For this review, take the finished solid that the model builds, in its own axes (mm). A direction names the side the tool comes from. Round coordinates to 2 decimals unless told otherwise and drop trailing zeros. Write each loop counter-clockwise with the first axis right and the second up, starting at its lowest first coordinate (ties: lowest second). Pieces come first, ordered by that corner, then holes. Notation, with made-up numbers: (63, 1.5) -> (94, 1.5) arc R23 cw to (94, 24.5) -> close; hole circle Ø5 at (66, 72). An arc over 180 degrees is marked (long way). Answer in a Markdown table with one row per item. Add a question column.
```python
from build123d import *

# Parameters (mm, degrees)
F0_R     = 4.25
F0_R_2   = 2.6
F1_DEPTH = 8
F0_R_3   = 10.25
F0_R_4   = 1.6
F2_DEPTH = 8
F3_DEPTH = 8
F4_DEPTH = 8
F5_R     = 1.9
F6_DEPTH = 27


with BuildPart() as f1:
    # F0 (on Top) → F1 (new body)
    with BuildSketch(Plane.XY):
        Circle(F0_R)
        Circle(F0_R_2, mode=Mode.SUBTRACT)
    extrude(amount=F1_DEPTH)

    # F0 (on Top) → F2 (join)
    with BuildSketch(Plane.XY):
        Circle(F0_R_3)
        with Locations((0, -7)):
            Circle(F0_R_2, mode=Mode.SUBTRACT)
        with Locations((-7, 0)):
            Circle(F0_R_4, mode=Mode.SUBTRACT)
        with Locations((-4.95, 4.9494949237)):
            Circle(F0_R_4, mode=Mode.SUBTRACT)
        Circle(F0_R, mode=Mode.SUBTRACT)
        with Locations((7, 0)):
            Circle(F0_R_4, mode=Mode.SUBTRACT)
        with Locations((4.95, 4.9494949237)):
            Circle(F0_R_4, mode=Mode.SUBTRACT)
        with Locations((0, 7)):
            Circle(F0_R_4, mode=Mode.SUBTRACT)
    extrude(amount=F2_DEPTH)

    # F0 (on Top) → F3 (join)
    with BuildSketch(Plane.XY):
        with BuildLine():
            ThreePointArc((11.5318049333, -3.3192581973), (11.8823747458, -1.6760579943), (12, 0))
            ThreePointArc((12, 0), (11.8823747458, 1.6760579943), (11.5318049333, 3.3192581973))
            ThreePointArc((11.5318049333, 3.3192581973), (8.3601945025, 8.6085508583), (2.9803472847, 11.6240066269))
            ThreePointArc((2.9803472847, 11.6240066269), (0, 12), (-2.9803472847, 11.6240066269))
            ThreePointArc((-2.9803472847, 11.6240066269), (-8.3601945025, 8.6085508583), (-11.5318049333, 3.3192581973))
            ThreePointArc((-11.5318049333, 3.3192581973), (-12, 0), (-11.5318049333, -3.3192581973))
            ThreePointArc((-11.5318049333, -3.3192581973), (-8.3601945025, -8.6085508583), (-2.9803472847, -11.6240066269))
            ThreePointArc((-2.9803472847, -11.6240066269), (0, -12), (2.9803472847, -11.6240066269))
            ThreePointArc((2.9803472847, -11.6240066269), (8.3601945025, -8.6085508583), (11.5318049333, -3.3192581973))
        make_face()
        Circle(F0_R_3, mode=Mode.SUBTRACT)
        with BuildLine():
            ThreePointArc((2.9803472847, 11.6240066269), (8.3601945025, 8.6085508583), (11.5318049333, 3.3192581973))
            Line((11.5318049333, 3.3192581973), (12.9980264072, 3.6470960391))
            ThreePointArc((12.9980264072, 3.6470960391), (9.5433558507, 9.5485265412), (3.6400549446, 13))
            Line((3.6400549446, 13), (3.3579982004, 13))
            Line((3.3579982004, 13), (2.9803472847, 11.6240066269))
        make_face()
        with BuildLine():
            ThreePointArc((-2.9803472847, 11.6240066269), (0, 12), (2.9803472847, 11.6240066269))
            Line((2.9803472847, 11.6240066269), (3.3579982004, 13))
            Line((3.3579982004, 13), (-3.3579982004, 13))
            Line((-3.3579982004, 13), (-2.9803472847, 11.6240066269))
        make_face()
        with BuildLine():
            ThreePointArc((3.6400549446, 13), (9.5433558507, 9.5485265412), (12.9980264072, 3.6470960391))
            ThreePointArc((12.9980264072, 3.6470960391), (13.3739178347, 1.8407394578), (13.5, 0))
            ThreePointArc((13.5, 0), (13.3739178347, -1.8407394578), (12.9980264072, -3.6470960391))
            ThreePointArc((12.9980264072, -3.6470960391), (9.5433558507, -9.5485265412), (3.6400549446, -13))
            Line((3.6400549446, -13), (16.5, -13))
            Line((16.5, -13), (16.5, 13))
            Line((16.5, 13), (3.6400549446, 13))
        make_face()
        with BuildLine():
            ThreePointArc((11.5318049333, 3.3192581973), (11.8823747458, 1.6760579943), (12, 0))
            ThreePointArc((12, 0), (11.8823747458, -1.6760579943), (11.5318049333, -3.3192581973))
            Line((11.5318049333, -3.3192581973), (12.9980264072, -3.6470960391))
            ThreePointArc((12.9980264072, -3.6470960391), (13.3739178347, -1.8407394578), (13.5, 0))
            ThreePointArc((13.5, 0), (13.3739178347, 1.8407394578), (12.9980264072, 3.6470960391))
            Line((12.9980264072, 3.6470960391), (11.5318049333, 3.3192581973))
        make_face()
        with BuildLine():
            Line((12.9980264072, -3.6470960391), (11.5318049333, -3.3192581973))
            ThreePointArc((11.5318049333, -3.3192581973), (8.3601945025, -8.6085508583), (2.9803472847, -11.6240066269))
            Line((2.9803472847, -11.6240066269), (3.3579982004, -13))
            Line((3.3579982004, -13), (3.6400549446, -13))
            ThreePointArc((3.6400549446, -13), (9.5433558507, -9.5485265412), (12.9980264072, -3.6470960391))
        make_face()
        with BuildLine():
            Line((3.3579982004, -13), (2.9803472847, -11.6240066269))
            ThreePointArc((2.9803472847, -11.6240066269), (0, -12), (-2.9803472847, -11.6240066269))
            Line((-2.9803472847, -11.6240066269), (-3.3579982004, -13))
            Line((-3.3579982004, -13), (3.3579982004, -13))
        make_face()
        with BuildLine():
            Line((-3.3579982004, -13), (-2.9803472847, -11.6240066269))
            ThreePointArc((-2.9803472847, -11.6240066269), (-8.3601945025, -8.6085508583), (-11.5318049333, -3.3192581973))
            Line((-11.5318049333, -3.3192581973), (-12.9980264072, -3.6470960391))
            ThreePointArc((-12.9980264072, -3.6470960391), (-9.5433558507, -9.5485265412), (-3.6400549446, -13))
            Line((-3.6400549446, -13), (-3.3579982004, -13))
        make_face()
        with BuildLine():
            ThreePointArc((-12.9980264072, -3.6470960391), (-13.5, 0), (-12.9980264072, 3.6470960391))
            ThreePointArc((-12.9980264072, 3.6470960391), (-9.5433558507, 9.5485265412), (-3.6400549446, 13))
            Line((-3.6400549446, 13), (-16.5, 13))
            Line((-16.5, 13), (-16.5, -13))
            Line((-16.5, -13), (-3.6400549446, -13))
            ThreePointArc((-3.6400549446, -13), (-9.5433558507, -9.5485265412), (-12.9980264072, -3.6470960391))
        make_face()
        with BuildLine():
            ThreePointArc((-11.5318049333, -3.3192581973), (-12, 0), (-11.5318049333, 3.3192581973))
            Line((-11.5318049333, 3.3192581973), (-12.9980264072, 3.6470960391))
            ThreePointArc((-12.9980264072, 3.6470960391), (-13.5, 0), (-12.9980264072, -3.6470960391))
            Line((-12.9980264072, -3.6470960391), (-11.5318049333, -3.3192581973))
        make_face()
        with BuildLine():
            ThreePointArc((-11.5318049333, 3.3192581973), (-8.3601945025, 8.6085508583), (-2.9803472847, 11.6240066269))
            Line((-2.9803472847, 11.6240066269), (-3.3579982004, 13))
            Line((-3.3579982004, 13), (-3.6400549446, 13))
            ThreePointArc((-3.6400549446, 13), (-9.5433558507, 9.5485265412), (-12.9980264072, 3.6470960391))
            Line((-12.9980264072, 3.6470960391), (-11.5318049333, 3.3192581973))
        make_face()
    extrude(amount=F3_DEPTH)

    # F0 (on Top) → F4 (join, symmetric)
    with BuildSketch(Plane.XY):
        with BuildLine():
            Line((-3.3579982004, -13), (-2.9803472847, -11.6240066269))
            ThreePointArc((-2.9803472847, -11.6240066269), (-8.3601945025, -8.6085508583), (-11.5318049333, -3.3192581973))
            Line((-11.5318049333, -3.3192581973), (-12.9980264072, -3.6470960391))
            ThreePointArc((-12.9980264072, -3.6470960391), (-9.5433558507, -9.5485265412), (-3.6400549446, -13))
            Line((-3.6400549446, -13), (-3.3579982004, -13))
        make_face()
        with BuildLine():
            Line((12.9980264072, -3.6470960391), (11.5318049333, -3.3192581973))
            ThreePointArc((11.5318049333, -3.3192581973), (8.3601945025, -8.6085508583), (2.9803472847, -11.6240066269))
            Line((2.9803472847, -11.6240066269), (3.3579982004, -13))
            Line((3.3579982004, -13), (3.6400549446, -13))
            ThreePointArc((3.6400549446, -13), (9.5433558507, -9.5485265412), (12.9980264072, -3.6470960391))
        make_face()
        with BuildLine():
            ThreePointArc((2.9803472847, 11.6240066269), (8.3601945025, 8.6085508583), (11.5318049333, 3.3192581973))
            Line((11.5318049333, 3.3192581973), (12.9980264072, 3.6470960391))
            ThreePointArc((12.9980264072, 3.6470960391), (9.5433558507, 9.5485265412), (3.6400549446, 13))
            Line((3.6400549446, 13), (3.3579982004, 13))
            Line((3.3579982004, 13), (2.9803472847, 11.6240066269))
        make_face()
        with BuildLine():
            ThreePointArc((-11.5318049333, 3.3192581973), (-8.3601945025, 8.6085508583), (-2.9803472847, 11.6240066269))
            Line((-2.9803472847, 11.6240066269), (-3.3579982004, 13))
            Line((-3.3579982004, 13), (-3.6400549446, 13))
            ThreePointArc((-3.6400549446, 13), (-9.5433558507, 9.5485265412), (-12.9980264072, 3.6470960391))
            Line((-12.9980264072, 3.6470960391), (-11.5318049333, 3.3192581973))
        make_face()
        with BuildLine():
            Line((3.3579982004, -13), (2.9803472847, -11.6240066269))
            ThreePointArc((2.9803472847, -11.6240066269), (0, -12), (-2.9803472847, -11.6240066269))
            Line((-2.9803472847, -11.6240066269), (-3.3579982004, -13))
            Line((-3.3579982004, -13), (3.3579982004, -13))
        make_face()
        with BuildLine():
            ThreePointArc((-11.5318049333, -3.3192581973), (-12, 0), (-11.5318049333, 3.3192581973))
            Line((-11.5318049333, 3.3192581973), (-12.9980264072, 3.6470960391))
            ThreePointArc((-12.9980264072, 3.6470960391), (-13.5, 0), (-12.9980264072, -3.6470960391))
            Line((-12.9980264072, -3.6470960391), (-11.5318049333, -3.3192581973))
        make_face()
        with BuildLine():
            ThreePointArc((11.5318049333, 3.3192581973), (11.8823747458, 1.6760579943), (12, 0))
            ThreePointArc((12, 0), (11.8823747458, -1.6760579943), (11.5318049333, -3.3192581973))
            Line((11.5318049333, -3.3192581973), (12.9980264072, -3.6470960391))
            ThreePointArc((12.9980264072, -3.6470960391), (13.3739178347, -1.8407394578), (13.5, 0))
            ThreePointArc((13.5, 0), (13.3739178347, 1.8407394578), (12.9980264072, 3.6470960391))
            Line((12.9980264072, 3.6470960391), (11.5318049333, 3.3192581973))
        make_face()
        with BuildLine():
            ThreePointArc((-2.9803472847, 11.6240066269), (0, 12), (2.9803472847, 11.6240066269))
            Line((2.9803472847, 11.6240066269), (3.3579982004, 13))
            Line((3.3579982004, 13), (-3.3579982004, 13))
            Line((-3.3579982004, 13), (-2.9803472847, 11.6240066269))
        make_face()
    extrude(amount=F4_DEPTH, both=True)

    # F5 (on face) → F6 (cut)
    with BuildSketch(Plane.XZ.offset(13)):
        with Locations((-14, 4)):
            Circle(F5_R)
        with Locations((14, 4)):
            Circle(F5_R)
    extrude(amount=-F6_DEPTH, mode=Mode.SUBTRACT)


solid = f1.part
```
1. We need section D-D (x = 7). Write out the cut boundary in (y, z).
2. For L1, parallel to Z at x = -14, y = -6.5; L2, parallel to X at y = -11, z = 4.5; L3, parallel to X at y = 5.25, z = 3.25, list the stretches that pass through material, from the lowest coordinate up. Write a range as [from, to].
3. We need section A-A (z = 4.5). Count the separate pieces of the cut face and the enclosed holes in it, plus the area to 3 significant figures.
4. Tool access review of faces 5 (the flat face through (14, 0, 0)), 6 (the flat face through (2, -2, 0)), 7 (the flat face through (-14, 0, 0)): name each direction out of +Z, -Z, +X, -X, +Y, -Y from which nothing blocks a thin tool from reaching the whole face with its end or side.
5. We need section C-C (y = 7). Write out the cut boundary in (x, z).
6. Clearance check with flat-ended pins moving along their axes: pin 1 Ø2.5 at (x, y) = (0, 7) entering from +Z; pin 2 Ø7 at (x, y) = (1, 4.5) entering from -Z; pin 3 Ø4 at (y, z) = (5, -3) entering from -X. State where each tip first meets the part, or that it passes through.
7. The part is to be moulded in two halves that separate along X. For faces 1 (the flat face through (0, 13, 2)), 2 (the flat face through (16.5, 0, 4)), 3 (the cylindrical face through (-0.338, 2.578, 3.944)), 4 (the flat face through (-16.5, 0, 4)), say which applies: pulls with the +X half, pulls with the -X half, needs draft (parallel to the pull), parting line crosses it, or undercut.
8. We need section B-B (x = 0). Write out the cut boundary in (y, z).
Response:
| question | item | result |
|---|---|---|
| 1 | outline | (-13, 0) -> (-11.54, 0) -> (-11.54, -8) -> (-9.75, -8) -> (-9.75, 0) -> (-1.6, 0) -> (-1.6, 8) -> (-13, 8) -> close; (1.6, 0) -> (9.75, 0) -> (9.75, -8) -> (11.54, -8) -> (11.54, 0) -> (13, 0) -> (13, 8) -> (1.6, 8) -> close |
| 2 | L1 | [0, 2.1], [5.9, 8] |
| 2 | L2 | [-16.5, -15.83], [-12.17, 12.17], [15.83, 16.5] |
| 2 | L3 | [-16.5, -15.75], [-12.25, -6.52], [-3.38, 3.38], [6.52, 12.25], [15.75, 16.5] |
| 3 | separate pieces | 3 |
| 3 | enclosed holes | 7 |
| 3 | area | 585 mm2 |
| 4 | face 5 | -Z, +X |
| 4 | face 6 | -Z |
| 4 | face 7 | -Z, -X |
| 5 | outline | (-16.5, 0) -> (-11.54, 0) -> (-11.54, -8) -> (-9.75, -8) -> (-9.75, 0) -> (-1.6, 0) -> (-1.6, 8) -> (-16.5, 8) -> close; (1.6, 0) -> (9.75, 0) -> (9.75, -8) -> (11.54, -8) -> (11.54, 0) -> (16.5, 0) -> (16.5, 8) -> (1.6, 8) -> close; hole circle Ø3.8 at (-14, 4); hole circle Ø3.8 at (14, 4) |
| 6 | pin 1 | through |
| 6 | pin 2 | z = 0 |
| 6 | pin 3 | x = -13.16 |
| 7 | face 1 | needs draft |
| 7 | face 2 | pulls with the +X half |
| 7 | face 3 | undercut |
| 7 | face 4 | pulls with the -X half |
| 8 | outline | (-13, -8) -> (-12, -8) -> (-12, 0) -> (-9.6, 0) -> (-9.6, 8) -> (-13, 8) -> close; (-4.4, 0) -> (-2.6, 0) -> (-2.6, 8) -> (-4.4, 8) -> close; (2.6, 0) -> (5.4, 0) -> (5.4, 8) -> (2.6, 8) -> close; (8.6, 0) -> (12, 0) -> (12, -8) -> (13, -8) -> (13, 8) -> (8.6, 8) -> close |
